Source: three-view drawing plus pictorial views. Frame: mm from the lowest corner of the part. A direction names the side the tool comes from. Give positions to 0.01 mm unless a question says otherwise; leave off trailing zeros. Write each loop counter-clockwise with the first axis right and the second up, starting at its lowest first coordinate (ties: lowest second). Pieces come first, ordered by that corner, then holes. Notation, with made-up numbers: (-15, -14.75) -> (22, -14.75) arc R24 ccw to (22, 5.25) -> close; hole circle Ø10 at (74.5, 74). An arc over 180 degrees is marked (long way). Answer in a Markdown table with one row per item. Add a question column.
Item 1: Section query B-B on x = 348. Output: boundary loops of the cut face in (y, z), plus the area to 3 significant figures.
Item 2: Draft query along Z for the marked faces 1, 2 and 3. Return one class per face: +Z half, -Z half, draft (parallel to the pull), parting line (faces both ways), or undercut.
Item 3: Section query D-D on z = 375. Output: boundary loops of the cut face in (x, y).
Item 4: Material intervals for probe 1 along Z at (x, y) = (153.5, 392); probe 2 along Y at (x, z) = (59.5, 32); probe 3 along Z at (x, y) = (61.5, 557), sorted ascending. Write a range as from..to.
Item 5: First-contact query: P1, Ø6, axis at x = 264.5, y = 130, coming from the -Z side; P2, Ø8, axis at x = 159, y = 343, coming from the +Z side. Flat tips, straight axial feed; report the tip coordinate or a pass-through.
Item 6: Section query A-A on y = 515. Output: boundary loops of the cut face in (x, z), plus the area to 3 significant figures.
Item 7: Access query for the marked faces 4, 5, 6 and 7. Directions: +Z, -Z, +X, -X, +Y, -Y. A direction counts if a zero-diameter tool reaches every point of the face in a straight line with its end or side. Return the directions, or none.
Item 8: Section query C-C on y = 613. Output: boundary loops of the cut face in (x, z), plus the area to 3 significant figures.
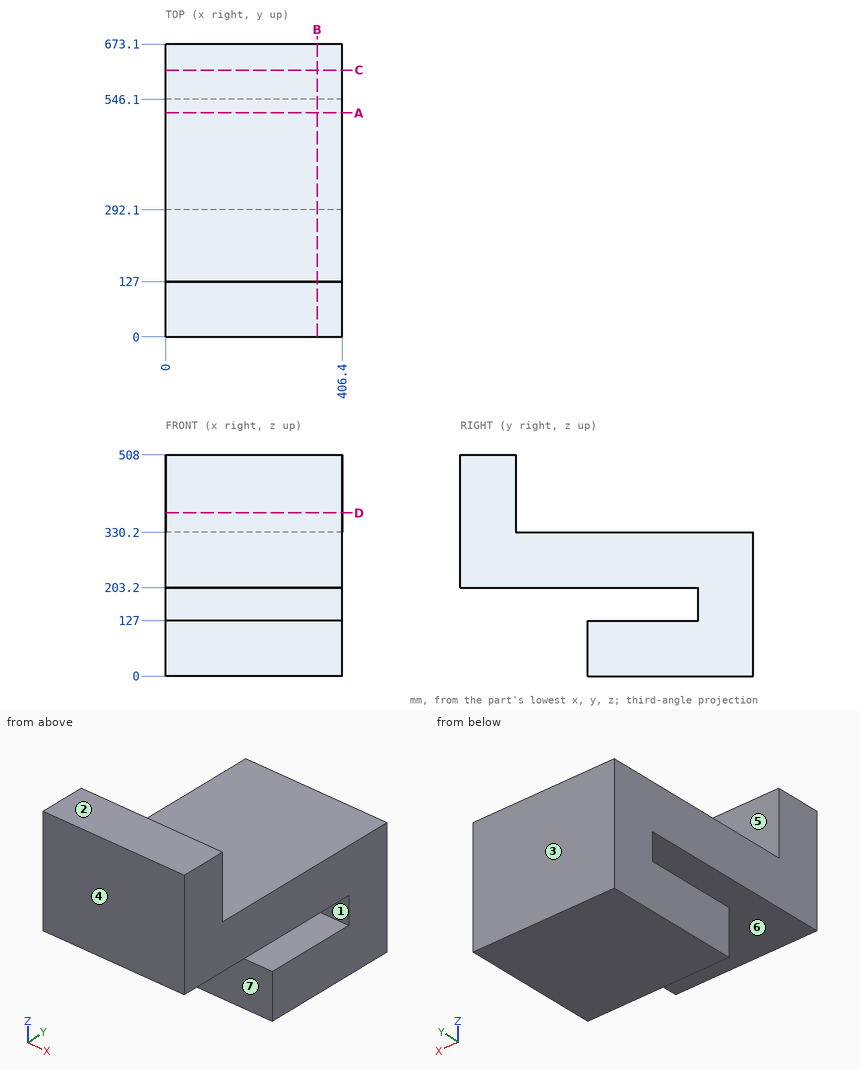
Findings below:
| question | item | result |
|---|---|---|
| 1 | outline | (0, 203.2) -> (546.1, 203.2) -> (546.1, 127) -> (292.1, 127) -> (292.1, 0) -> (673.1, 0) -> (673.1, 330.2) -> (127, 330.2) -> (127, 508) -> (0, 508) -> close |
| 1 | area | 166,000 mm^2 |
| 2 | face 1 | undercut |
| 2 | face 2 | +Z half |
| 2 | face 3 | draft |
| 3 | outline | (0, 0) -> (406.4, 0) -> (406.4, 127) -> (0, 127) -> close |
| 4 | probe 1 | z = 0..127, 203.2..330.2 |
| 4 | probe 2 | y = 292.1..673.1 |
| 4 | probe 3 | z = 0..330.2 |
| 5 | P1 | stops at z = 203.2 |
| 5 | P2 | stops at z = 330.2 |
| 6 | outline | (0, 0) -> (406.4, 0) -> (406.4, 127) -> (0, 127) -> close; (0, 203.2) -> (406.4, 203.2) -> (406.4, 330.2) -> (0, 330.2) -> close |
| 6 | area | 103,000 mm^2 |
| 7 | face 4 | +Z, -Z, +X, -X, -Y |
| 7 | face 5 | +Z, +X, -X, +Y |
| 7 | face 6 | +X, -X, -Y |
| 7 | face 7 | -Z, +X, -X, -Y |
| 8 | outline | (0, 0) -> (406.4, 0) -> (406.4, 330.2) -> (0, 330.2) -> close |
| 8 | area | 134,000 mm^2 |
